from build123d import *

# Parameters (mm, degrees)
SKETCH2_R          = 9.65
CUT_EXTRUDE1_DEPTH = 1.4
CUT_EXTRUDE2_START = -1.4
SKETCH3_R          = 9.65
CUT_EXTRUDE2_DEPTH = 1.4
CHAMFER1_SIZE      = 0.25


with BuildPart() as part:
    # Sketch1 → Revolve1 (revolve)
    with BuildSketch(Plane(origin=(0, 0, 0), x_dir=(0, 0, -1), z_dir=(1, 0, 0)), mode=Mode.PRIVATE) as revolve1_sk:
        with BuildLine():
            Line((-6.25, 17), (-7.25, 17))
            Line((-7.25, 17), (-7.25, 8.65))
            Line((-7.25, 8.65), (7.25, 8.65))
            Line((7.25, 8.65), (7.25, 17))
            Line((7.25, 17), (6.25, 17))
            ThreePointArc((6.25, 17), (0, 10.75), (-6.25, 17))
        make_face()
    revolve(revolve1_sk.sketch.rotate(Axis((0, 0, 64.980952982), (0, 0, -1)), 90), axis=Axis((0, 0, 64.980952982), (0, 0, -1)))

    # Sketch2 → Cut-Extrude1 (cut)
    with BuildSketch(Plane(origin=(0, 0, -7.25), x_dir=(-1, 0, 0), z_dir=(0, 0, -1))):
        Circle(SKETCH2_R)
    extrude(amount=-CUT_EXTRUDE1_DEPTH, mode=Mode.SUBTRACT)

    # Sketch3 → Cut-Extrude2 (cut)
    with BuildSketch(Plane.XY.offset(7.25).offset(CUT_EXTRUDE2_START)):
        with Locations(Location((0, 0, 0), (0, 0, 180))):
            Circle(SKETCH3_R)
    extrude(amount=CUT_EXTRUDE2_DEPTH, mode=Mode.SUBTRACT)

    # Chamfer1
    chamfer1_edges = [part.edges().sort_by_distance(p)[0] for p in [
        (9.65, 0, -7.25),
        (-8.65, 0, -5.85),
        (9.65, 0, 7.25),
        (-8.65, 0, 5.85),
    ]]
    chamfer(chamfer1_edges, length=CHAMFER1_SIZE)


solid = part.part
Here's how the part is built. I have some questions about the finished solid (model axes, mm). A direction names the side the tool comes from. Give positions to 0.01 mm unless a question says otherwise; leave off trailing zeros. Write each loop counter-clockwise with the first axis right and the second up, starting at its lowest first coordinate (ties: lowest second). Pieces come first, ordered by that corner, then holes. Notation, with made-up numbers: (-31, 45) -> (-1, 45) arc R5 ccw to (-1, 52) -> close; hole circle Ø2 at (85.25, -2). An arc over 180 degrees is marked (long way). Use one line per item in the form item = value. Start each with the question number.
1. On a 3-axis mill with a long thin cutter (end or side, diameter ignored), from which of +Z, -Z, +X, -X, +Y, -Y can I reach the whole of each face in a straight line? I mean faces 1 (the face through (-9, -3, -5.85)), 2 (the face through (-9.204, -2.899, 6.417)), 3 (the face through (8.25, -2.6, -0.08)). Say none if no direction works.
2. Imagine slicing it at C-C on z = 0. List the corners of the cut face in (x, y) for me, plus the area to 3 significant figures.
3. If I drill on L1, parallel to Y at x = 0, z = -6.6; L2, parallel to X at y = -6, z = -4; L3, parallel to Z at x = 7.5, y = -10.5, over which ranges is the centre line in solid material (lowest first)?
4. Thinking about a two-plate mould opening in Y: for faces 4 (the face through (-2.213, -16.855, 6.757)), 5 (the face through (-7.3, 7.3, -7.25)), 6 (the face through (-9.204, 2.899, -6.433)), which applies, +Y half, -Y half, draft (parallel to the pull), parting line (faces both ways), or undercut?
5. Imagine slicing it at D-D on z = 4.5. List the corners of the cut face in (x, y) for me.
6. Imagine slicing it at A-A on x = 0. List the corners of the cut face in (y, z) for me, plus the area to 3 significant figures.
7. Will these pins go through, and if not, where does the flat tip stop? pin 1 Ø15.5 at (x, y) = (0, 0) entering from +Z; pin 2 Ø1 at (y, z) = (-10, -0.5) entering from -X; pin 3 Ø4 at (y, z) = (-2.5, 4.5) entering from -X; pin 4 Ø1 at (x, z) = (-2, 4) entering from +Y.
Entries:
q1.face_1 = -Z
q1.face_2 = +Z
q1.face_3 = +Z, -Z
q2.outline = circle Ø21.5 at (0, 0); hole circle Ø17.3 at (0, 0)
q2.area = 128 mm²
q3.L1 = -17 to -9.65, 9.65 to 17
q3.L2 = -10.62 to -6.23, 6.23 to 10.62
q3.L3 = -7.25 to -4.72, 4.72 to 7.25
q4.face_4 = parting line
q4.face_5 = draft
q4.face_6 = undercut
q5.outline = circle Ø25.33 at (0, 0); hole circle Ø17.3 at (0, 0)
q6.outline = (-17, -7.25) -> (-9.9, -7.25) -> (-9.65, -7) -> (-9.65, -5.85) -> (-8.9, -5.85) -> (-8.65, -5.6) -> (-8.65, 5.6) -> (-8.9, 5.85) -> (-9.65, 5.85) -> (-9.65, 7) -> (-9.9, 7.25) -> (-17, 7.25) -> (-17, 6.25) arc R6.25 cw to (-17, -6.25) -> close; (8.65, -5.6) -> (8.9, -5.85) -> (9.65, -5.85) -> (9.65, -7) -> (9.9, -7.25) -> (17, -7.25) -> (17, -6.25) arc R6.25 cw to (17, 6.25) -> (17, 7.25) -> (9.9, 7.25) -> (9.65, 7) -> (9.65, 5.85) -> (8.9, 5.85) -> (8.65, 5.6) -> close
q6.area = 114 mm²
q7.pin_1 = through
q7.pin_2 = -5.08
q7.pin_3 = -16.93
q7.pin_4 = 12.51
